from build123d import *

# Parameters (mm, degrees)
F1_DEPTH = 111.651853
F2_R     = 46.360337
F3_DEPTH = 307.816686


with BuildPart() as f1:
    # F0 (on Front) → F1 (new body)
    with BuildSketch(Plane.XZ):
        Polygon((0, 0), (141.16028, 0), (141.16028, 84.286302), (88.496365, 144.964725), align=None)
    extrude(amount=F1_DEPTH)

    # F2 (on face) → F3 (join)
    with BuildSketch(Plane(origin=(0, 0, 0), x_dir=(-1, 0, 0), z_dir=(0, 1, 0))):
        with Locations((-93.247063, 41.50847)):
            Circle(F2_R)
    extrude(amount=F3_DEPTH)


solid = f1.part
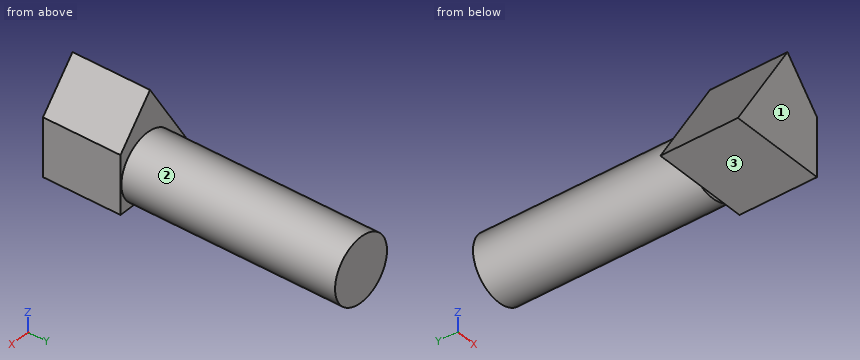
Model file for the job. Use its own axes, mm. Face numbers are marked on the shaded views. A direction names the side the tool comes from. Round coordinates to 2 decimals unless told otherwise and drop trailing zeros. Order: outer loops, then holes, each group sorted by start corner. A loop starts at its lowest first (then second) coordinate and runs counter-clockwise, first axis right, second up. Notation, with made-up numbers: M -10,8 L 36,8 A35 cw 36,43 Z; hole C 60,37.25 d7. An arc over 180 degrees is marked long. Write each question's results on one line, items separated by ' | '. Start each with the question number.
(1) Which spindle directions (+Z, -Z, +X, -X, +Y, -Y) get a long thin tool onto all of the face, cutting with end or side? Do the marked faces 1, 2 and 3. Say none if no direction does.
(2) Saw through at A-A, the plane z = 50. Give the cut face in (x, y), then the cut area to 3 significant figures.
(3) Drop flat-ended pins along their axis: pin 1 (4 mm diameter, centred on x = 100.5, z = -3, fed in from -Y); pin 2 (2 mm diameter, centred on y = 134, z = 23, fed in from -X); pin 3 (4 mm diameter, centred on x = 109, z = 91.5, fed in from +Y). Give the stop position or say it passes through.
(4) Saw through at B-B, the plane x = 66. Give the cut face in (y, z).
(5) Saw through at D-D, the plane y = 257.5. Give the cut face in (x, z), then the cut area to 3 significant figures.
(6) Probe probe 1 along Y at (x, z) = (42, 37.5); probe 2 along X at (y, z) = (-7, 119); probe 3 along X at (y, z) = (77.5, 38). List the from-to ranges inside material, lowest first. Write a range as from..to.
(7) Saw through at C-C, the plane y = -54.5. Give the cut face in (x, z).
Established:
1) face 1: +Z, -Z, +X, -X, -Y | face 2: +Y | face 3: -Z, +X, -X, -Y
2) outline: M 30.52,-111.65 L 141.16,-111.65 L 141.16,0 L 138.82,0 L 138.82,307.82 L 47.67,307.82 L 47.67,0 L 30.52,0 Z | area: 40,400 mm^2
3) pin 1: stops at y = 0 | pin 2: stops at x = 50.32 | pin 3: stops at y = 0
4) outline: M -111.65,0 L 0,0 L 0,4 L 307.82,4 L 307.82,79.02 L 0,79.02 L 0,108.11 L -111.65,108.11 Z
5) outline: C 93.25,41.51 d92.72 | area: 6,750 mm^2
6) probe 1: y = -111.65..0 | probe 2: x = 72.65..111.03 | probe 3: x = 47.02..139.47
7) outline: M 0,0 L 141.16,0 L 141.16,84.29 L 88.5,144.96 Z
